from build123d import *

# Parameters (mm, degrees)
F1_DEPTH = 4
F2_R     = 3.99999


# Not quite as in the source:
# - a fillet or chamfer is up to 0.001 mm smaller than in the source, because OpenCascade refuses the exact size
# - ends of sketch curves that miss each other by under 0.0002 mm in the source are joined
# - a feature names something its author has since deleted; it is built from what else it names


with BuildPart() as f1:
    # F0 (on Front) → F1 (new body, symmetric)
    with BuildSketch(Plane.XZ):
        Polygon((-14.732436277, -7.7009890229), (-14.732436277, 0), (-22.7324279615, -0.0115346295), (-22.721270651, -7.7498318101), align=None)
        Polygon((-22.721270651, -7.7498318101), (-22.7324279615, -0.0115346295), (-30.732419646, -0.0230692591), (-30.7212084456, -7.7987424823), align=None)
        Polygon((-30.7212084456, -7.7987424823), (-30.732419646, -0.0230692591), (-38.7324113305, -0.0346038886), (-38.7211462402, -7.8476531545), align=None)
        Polygon((-38.7211462402, -7.8476531545), (-38.7324113305, -0.0346038886), (-46.732403015, -0.0461385181), (-46.6844078154, -7.8963395926), align=None)
        Polygon((-46.6844078154, -7.8963395926), (-46.732403015, -0.0461385181), (-54.7323946996, -0.0576731477), (-54.7210218294, -7.9454744989), align=None)
        Polygon((-54.7210218294, -7.9454744989), (-54.7323946996, -0.0576731477), (-62.7323863841, -0.0692077772), (-62.7208598391, -7.994384561), align=None)
        Polygon((-62.7208598391, -7.994384561), (-62.7322865984, -0.0692076333), (-70.7323780686, -0.0807424068), (-70.7208974186, -8.0432958433), align=None)
        Polygon((-70.7208974186, -8.0432958433), (-70.7323780686, -0.0807424068), (-78.7323697531, -0.0922770363), (-78.7323697531, -8.0922770363), align=None)
    extrude(amount=F1_DEPTH, both=True)

    # F2 (radius 4 in the source; OpenCascade refuses exactly that, so slightly less here)
    f2_edges = [f1.edges().sort_by_distance(p)[0] for p in [
        (-78.73237, 4, -4.092277),
        (-78.73237, -4, -4.092277),
        (-14.732436, 4, -3.850495),
        (-14.732436, -4, -3.850495),
    ]]
    fillet(f2_edges, radius=F2_R)


solid = f1.part
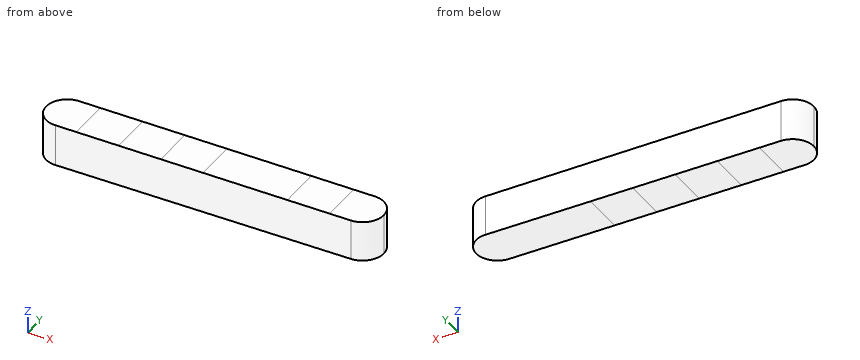
CAD build for the part. Positions are in the model's coordinates, mm. Give positions to 0.01 mm unless a question says otherwise; leave off trailing zeros. Write each loop counter-clockwise with the first axis right and the second up, starting at its lowest first coordinate (ties: lowest second). Pieces come first, ordered by that corner, then holes. Notation, with made-up numbers: M -26.75,9 L 12.25,9 A26 cw 12.25,30 Z; hole C 3.5,80 d6. An arc over 180 degrees is marked long. Put each result on its own line as item: value. Start each with the question number.
(1) Flat gauge pins, fed straight in: pin 1 Ø1.5 at (x, y) = (-53, -0.5) entering from -Z; pin 2 Ø1 at (x, y) = (-67.5, -1) entering from +Z. Where does each tip first touch, or does it go through?
(2) Probe L1, parallel to Z at x = -19.5, y = -3.5; L2, parallel to Z at x = -54.5, y = 0; L3, parallel to X at y = 0.25, z = -6.5. List the from-to ranges inside material, lowest first.
(3) Band-saw the part on A-A, the plane y = 2. Write the cut outline in (x, z).
(4) Band-saw the part on D-D, the plane y = -2.75. Write the cut outline in (x, z), and give its area (3 significant figures).
(5) Band-saw the part on C-C, the plane x = -21. Write the cut outline in (y, z).
Response values:
1. pin 1: stops at z = -7.94
1. pin 2: stops at z = -0.08
2. L1: z = -7.73 to -0.01
2. L2: z = -7.94 to -0.06
2. L3: x = -78.72 to -14.74
3. outline: M -78.2,-8.09 L -15.27,-7.7 L -15.27,0 L -78.2,-0.09 Z
4. outline: M -77.64,-8.09 L -15.83,-7.71 L -15.83,0 L -77.64,-0.09 Z
4. area: 485 mm2
5. outline: M -4,-7.74 L 4,-7.74 L 4,-0.01 L -4,-0.01 Z
